from build123d import *

# Parameters (mm, degrees)
F0_W     = 53
F0_H     = 9
F0_R     = 2.25
F1_DEPTH = 1.2
F2_R     = 1
F3_SIZE  = 0.5


with BuildPart() as f1:
    # F0 (on Top) → F1 (new body)
    with BuildSketch(Plane.XY):
        Rectangle(F0_W, F0_H)
        with Locations((-21.5, 0)):
            Circle(F0_R, mode=Mode.SUBTRACT)
        with BuildLine():
            Line((3, -2.25), (-2, -2.25))
            ThreePointArc((-2, -2.25), (-4.25, 0), (-2, 2.25))
            Line((-2, 2.25), (3, 2.25))
            ThreePointArc((3, 2.25), (5.25, 0), (3, -2.25))
        make_face(mode=Mode.SUBTRACT)
        with BuildLine():
            Line((21.5, -2.25), (16.5, -2.25))
            ThreePointArc((16.5, -2.25), (14.25, 0), (16.5, 2.25))
            Line((16.5, 2.25), (21.5, 2.25))
            ThreePointArc((21.5, 2.25), (23.75, 0), (21.5, -2.25))
        make_face(mode=Mode.SUBTRACT)
    extrude(amount=F1_DEPTH)

    # F2
    f2_edges = [f1.edges().sort_by_distance(p)[0] for p in [
        (-26.5, -4.5, 0.6),
        (-26.5, 4.5, 0.6),
        (26.5, -4.5, 0.6),
        (26.5, 4.5, 0.6),
    ]]
    fillet(f2_edges, radius=F2_R)

    # F3
    f3_edges = [f1.edges().sort_by_distance(p)[0] for p in [
        (-23.75, 0, 1.2),
        (-4.25, 0, 1.2),
        (14.25, 0, 1.2),
    ]]
    chamfer(f3_edges, length=F3_SIZE)


solid = f1.part
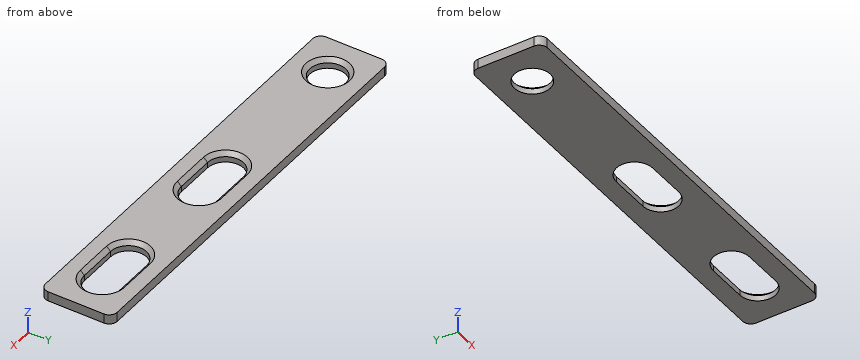
Can you work these out from the model? Positions are in its coordinate system, mm. Round coordinates to 2 decimals unless told otherwise and drop trailing zeros. Write each loop counter-clockwise with the first axis right and the second up, starting at its lowest first coordinate (ties: lowest second). Pieces come first, ordered by that corner, then holes. Notation, with made-up numbers: (-35, 24) - (20, 24) arc R8 ccw to (20, 34) - close; hole circle Ø5 at (53, 17). An arc over 180 degrees is marked (long way). Write each question's results on one line, items separated by ' | '. Start each with the question number.
1) Suppose I cut it at A-A (x = -21.5). List the corners of the cut face in (y, z) for me.
2) For pin 1 Ø2 at (x, y) = (0, -1.5) entering from -Z, with a flat end and sliding along its axis, tell me the tip position at first contact or that it passes through.
3) Please list where these lines run through material, in increasing order: line 1 (Y direction, x = -21.5, z = 0.55); line 2 (X direction, y = -1.5, z = 1); line 3 (X direction, y = -1.25, z = 0.55).
4) Suppose I cut it at C-C (z = 0.3). List the corners of the cut face in (x, y) for me, and give its area (3 significant figures).
5) Suppose I cut it at B-B (y = 0). List the corners of the cut face in (x, z) for me, and give its area (4 significant figures).
Here are the results:
1) outline: (-4.5, 0) - (-2.25, 0) - (-2.25, 0.7) - (-2.75, 1.2) - (-4.5, 1.2) - close; (2.25, 0) - (4.5, 0) - (4.5, 1.2) - (2.75, 1.2) - (2.25, 0.7) - close
2) pin 1: stops at z = 0
3) line 1: y = -4.5 to -2.25, 2.25 to 4.5 | line 2: x = -26.5 to -23.56, -19.44 to -4.06, 5.06 to 14.44, 23.56 to 26.5 | line 3: x = -26.5 to -23.37, -19.63 to -3.87, 4.87 to 14.63, 23.37 to 26.5
4) outline: (-26.5, -3.5) arc R1 ccw to (-25.5, -4.5) - (25.5, -4.5) arc R1 ccw to (26.5, -3.5) - (26.5, 3.5) arc R1 ccw to (25.5, 4.5) - (-25.5, 4.5) arc R1 ccw to (-26.5, 3.5) - close; hole circle Ø4.5 at (-21.5, 0); hole (-2, -2.25) - (3, -2.25) arc R2.25 ccw to (3, 2.25) - (-2, 2.25) arc R2.25 ccw to start; hole (16.5, -2.25) - (21.5, -2.25) arc R2.25 ccw to (21.5, 2.25) - (16.5, 2.25) arc R2.25 ccw to start | area: 383 mm2
5) outline: (-26.5, 0) - (-23.75, 0) - (-23.75, 0.7) - (-24.25, 1.2) - (-26.5, 1.2) - close; (-19.25, 0) - (-4.25, 0) - (-4.25, 0.7) - (-4.75, 1.2) - (-18.75, 1.2) - (-19.25, 0.7) - close; (5.25, 0) - (14.25, 0) - (14.25, 0.7) - (13.75, 1.2) - (5.75, 1.2) - (5.25, 0.7) - close; (23.75, 0) - (26.5, 0) - (26.5, 1.2) - (24.25, 1.2) - (23.75, 0.7) - close | area: 34.65 mm2
